Could you check a few things on this model? Use its own coordinates, in mm. A direction names the side the tool comes from. Give positions to 0.01 mm unless a question says otherwise; leave off trailing zeros. Loops run counter-clockwise (first coordinate to the right, second up) from the corner with the lowest first, then second, coordinate; pieces in that order, holes last. Notation, with made-up numbers: M 55.5,-28.75 L 97.5,-28.75 A20 cw 97.5,9.25 Z; hole C -10.5,55 d3. An arc over 180 degrees is marked long. Answer in a Markdown table with one row per item. Add a question column.
1. If we section it at A-A on z = -11: List the corners of the cut face in (x, y) for me.
2. Thinking about a two-plate mould opening in X: for faces 4 (the flat face through (75, 5, -1)), 5 (the flat face through (-5, 5, -38)), 6 (the cylindrical face through (5.07, 4.93, -12.5)), which applies, released by +X, released by -X, zero draft, split by the parting line, or undercut?
3. If we section it at D-D on y = 2: Count the separate pieces of the cut face and the enclosed holes in it, then the cut area to 3 significant figures.
4. If we section it at B-B on x = 15: List the corners of the cut face in (y, z) for me, then the cut area to 3 significant figures.
5. I'm going to push flat-ended pins straight in: pin 1 Ø6 at (x, z) = (58.5, -28.5) entering from -Y; pin 2 Ø3 at (y, z) = (3, -38.5) entering from -X; pin 3 Ø0.9 at (y, z) = (4.5, -5) entering from +X; pin 4 Ø5 at (x, y) = (70, 6) entering from -Z. Where does each tip first touch, or does it pass through?
6. Which directions (+Z, -Z, +X, -X, +Y, -Y) give clear straight access to the entire face, cutting with the end or side of a thin tool? Please do faces 1 (the flat face through (25, 5, -6)), 2 (the flat face through (0, 5, -53)), 3 (the flat face through (55, 5, -32)).
7. I need wall thicknesses on line 1 along X through (y, z) = (2.5, -56); line 2 along Z through (x, y) = (25.5, 2.5); line 3 along X through (y, z) = (8.5, -38). Which ranges of each line are inside material? Lowest first, please. Write a range as from..to.
8. If we section it at C-C on x = 5: List the corners of the cut face in (y, z) for me, then the cut area to 3 significant figures.
```python
from build123d import *

# Parameters (mm, degrees)
SKETCH1_R           = 1.5
BOSS_EXTRUDE1_DEPTH = 10


with BuildPart() as part:
    # Sketch1 → Boss-Extrude1 (new body)
    with BuildSketch(Plane(origin=(0, 0, 0), x_dir=(1, 0, 0), z_dir=(0, 1, 0))):
        with BuildLine():
            Line((55, 4), (55, 60))
            ThreePointArc((55, 60), (54.707106781, 60.707106781), (54, 61))
            Line((54, 61), (1, 61))
            ThreePointArc((1, 61), (0.292893219, 60.707106781), (0, 60))
            Line((0, 60), (0, 46.362049935))
            ThreePointArc((0, 46.362049935), (-0.059728422, 46.021624671), (-0.23177872, 45.721865536))
            Line((-0.23177872, 45.721865536), (-4.76822128, 40.278134464))
            ThreePointArc((-4.76822128, 40.278134464), (-4.940271578, 39.978375329), (-5, 39.637950065))
            Line((-5, 39.637950065), (-5, 36))
            ThreePointArc((-5, 36), (-4.707106781, 35.292893219), (-4, 35))
            Line((-4, 35), (-3, 35))
            Line((-3, 35), (0, 38.6))
            Line((0, 38.6), (0, 6))
            Line((0, 6), (51, 6))
            ThreePointArc((51, 6), (51.707106781, 5.707106781), (52, 5))
            Line((52, 5), (52, 4))
            ThreePointArc((52, 4), (51.707106781, 3.292893219), (51, 3))
            Line((51, 3), (-0.5, 3))
            ThreePointArc((-0.5, 3), (-1.207106781, 3.292893219), (-1.5, 4))
            Line((-1.5, 4), (-1.5, 7))
            Line((-1.5, 7), (-8.947213595, 3.276393202))
            ThreePointArc((-8.947213595, 3.276393202), (-9.350650808, 2.907697123), (-9.5, 2.381966011))
            Line((-9.5, 2.381966011), (-9.5, 1))
            ThreePointArc((-9.5, 1), (-9.207106781, 0.292893219), (-8.5, 0))
            Line((-8.5, 0), (75, 0))
            Line((75, 0), (75, 3))
            Line((75, 3), (56, 3))
            ThreePointArc((56, 3), (55.292893219, 3.292893219), (55, 4))
        make_face()
        with Locations(Location((5, 56, 0), (0, 0, 270))):
            Circle(SKETCH1_R, mode=Mode.SUBTRACT)
        with Locations(Location((50, 56, 0), (0, 0, 270))):
            Circle(SKETCH1_R, mode=Mode.SUBTRACT)
        with Locations(Location((5, 11, 0), (0, 0, 270))):
            Circle(SKETCH1_R, mode=Mode.SUBTRACT)
        with Locations(Location((50, 11, 0), (0, 0, 270))):
            Circle(SKETCH1_R, mode=Mode.SUBTRACT)
    extrude(amount=BOSS_EXTRUDE1_DEPTH)


solid = part.part
```
Results:
| question | item | result |
|---|---|---|
| 1 | outline | M 0,0 L 3.5,0 L 3.5,10 L 0,10 Z; M 6.5,0 L 48.5,0 L 48.5,10 L 6.5,10 Z; M 51.5,0 L 55,0 L 55,10 L 51.5,10 Z |
| 2 | face 4 | released by +X |
| 2 | face 5 | released by -X |
| 2 | face 6 | undercut |
| 3 | separate pieces | 1 |
| 3 | enclosed holes | 4 |
| 3 | area | 3,310 mm2 |
| 4 | outline | M 0,-61 L 10,-61 L 10,-6 L 0,-6 Z; M 0,-3 L 10,-3 L 10,0 L 0,0 Z |
| 4 | area | 580 mm2 |
| 5 | pin 1 | through |
| 5 | pin 2 | x = -5 |
| 5 | pin 3 | x = 55 |
| 5 | pin 4 | z = -3 |
| 6 | face 1 | +Y, -Y |
| 6 | face 2 | -Z, -X, +Y, -Y |
| 6 | face 3 | -Z, +X, +Y, -Y |
| 7 | line 1 | 0..3.5, 6.5..48.5, 51.5..55 |
| 7 | line 2 | -61..-6, -3..0 |
| 7 | line 3 | -5..-0.5, 0..55 |
| 8 | outline | M 0,-61 L 10,-61 L 10,-57.5 L 0,-57.5 Z; M 0,-54.5 L 10,-54.5 L 10,-12.5 L 0,-12.5 Z; M 0,-9.5 L 10,-9.5 L 10,-6 L 0,-6 Z; M 0,-3 L 10,-3 L 10,0 L 0,0 Z |
| 8 | area | 520 mm2 |
